Geometry check sheet. Reference: drawing and pictorial views, mm from the part's lowest x, y, z. Round coordinates to 2 decimals unless told otherwise and drop trailing zeros. Put each result on its own line as item: value.
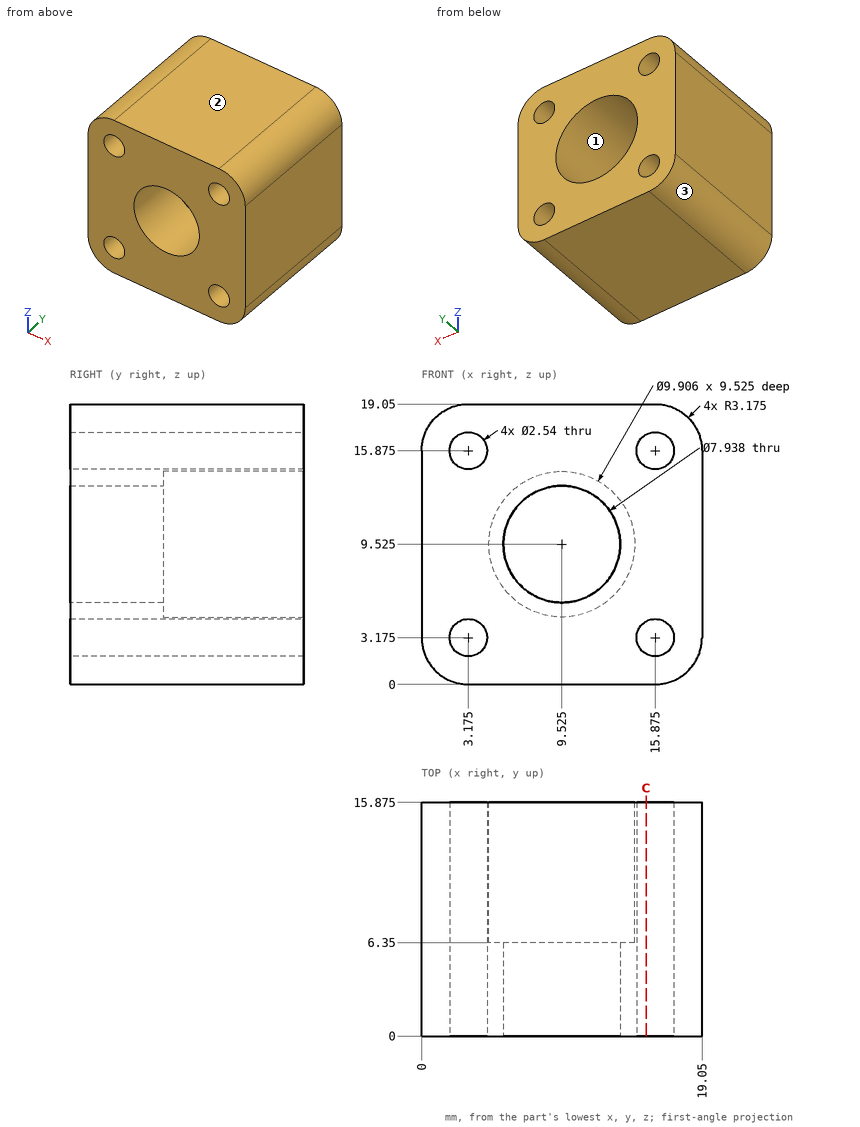
Item 1: Material ranges on line 1 along Z through (x, y) = (16, 9); line 2 along X through (y, z) = (1.75, 15.25); line 3 along Z through (x, y) = (9.75, 4.5), recorded low to high.
Geometry check:
line 1: 0 to 1.91, 4.44 to 14.61, 17.14 to 19.05
line 2: 0 to 2.07, 4.28 to 14.77, 16.98 to 19.05
line 3: 0 to 5.56, 13.49 to 19.05
Item 2: Release check for a two-part mould opening along Z. For the marked faces 1, 2 and 3 record: pulls with the +Z half, pulls with the -Z half, needs draft (parallel to the pull), parting line crosses it, or undercut.
Geometry check:
face 1: undercut
face 2: pulls with the +Z half
face 3: pulls with the -Z half
Item 3: Depth check by flat-ended pin: pin 1 Ø8 at (x, z) = (9, 9.5) entering from +Y. Enter the tip coordinate at first touch or a pass-through.
Geometry check:
pin 1: y = 6.35
Item 4: Sectioned sample at C-C, the plane x = 15.25. Give the number of separate pieces and of enclosed holes in the cut face, then the cut area to 3 significant figures.
Geometry check:
separate pieces: 3
enclosed holes: 0
area: 232 mm2
